The model under review builds one solid part; all positions refer to its coordinate system, in mm. A direction names the side the tool comes from. Give positions to 0.01 mm unless a question says otherwise; leave off trailing zeros. Order: outer loops, then holes, each group sorted by start corner. A loop starts at its lowest first (then second) coordinate and runs counter-clockwise, first axis right, second up. Notation, with made-up numbers: (40, -34) - (53, -34) arc R36 cw to (53, 3) - close; hole circle Ø1 at (-17.5, -38.75). An arc over 180 degrees is marked (long way). Use CSV: the item, a comma, the result in double quotes. Start each with the question number.
1. Take a section at A-A, the plane z = 31.5. State the section outline as (x, y) points, then the cut area to 3 significant figures.
2. Take a section at C-C, the plane x = -126.5. State the section outline as (y, z) points.
3. Machinability: for faces 5 (the flat face through (-102, 0, 10)), 6 (the flat face through (-152.89, 4, 31)), which of the approach directions +Z, -Z, +X, -X, +Y, -Y give a long, thin tool a straight path to every point of the face, cutting with its end or side? Answer none if there is none.
4. Draft analysis for pull direction X (two halves, no side actions). For faces 1 (the flat face through (-118, 10, 52)), 2 (the flat face through (-103, 4, 10.186)), 3 (the flat face through (-49.89, 5, 31)), 4 (the flat face through (-102, 9, 52)), state which applies: released by +X, released by -X, zero draft, split by the parting line, or undercut.
5. Take a section at B-B, the plane y = 6. State the section outline as (x, z) points, then the cut area to 3 significant figures.
6. To check wall thickness, follow line 1 (Z direction, x = -131, y = 3.75); line 2 (X direction, y = 0.5, z = 34). State the ranges of each line that lie inside material, in increasing order. Write a range as [from, to].
```python
from build123d import *

# Parameters (mm, degrees)
F0_W     = 104
F0_H     = 44
F0_W_2   = 100
F0_H_2   = 40
F1_DEPTH = 10
F2_T     = -1
F3_DEPTH = 25


with BuildPart() as f1:
    # F0 (on Front) → F1 (new body)
    with BuildSketch(Plane.XZ):
        with Locations((-101.889864, 31.185937)):
            Rectangle(F0_W, F0_H)
        with Locations((-101.889864, 31.185937)):
            Rectangle(F0_W_2, F0_H_2, mode=Mode.SUBTRACT)
        with Locations((-101.889864, 31.185937)):
            Rectangle(F0_W_2, F0_H_2)
    extrude(amount=-F1_DEPTH)

    # F2
    f2_openings = [f1.faces().sort_by_distance(p)[0] for p in [
        (-101.889864, 0, 31.185937),
    ]]
    offset(amount=F2_T, openings=f2_openings)

    # F0 (on Front) → F3 (cut)
    with BuildSketch(Plane.XZ):
        with Locations((-101.889864, 31.185937)):
            Rectangle(F0_W_2, F0_H_2)
    extrude(amount=-F3_DEPTH, mode=Mode.SUBTRACT)


solid = f1.part
```
Determined:
1,outline,"(-153.89, 0) - (-152.89, 0) - (-152.89, 9) - (-151.89, 9) - (-151.89, 10) - (-153.89, 10) - close; (-51.89, 9) - (-50.89, 9) - (-50.89, 0) - (-49.89, 0) - (-49.89, 10) - (-51.89, 10) - close"
1,area,"22.0 mm²"
2,outline,"(0, 9.19) - (10, 9.19) - (10, 11.19) - (9, 11.19) - (9, 10.19) - (0, 10.19) - close; (0, 52.19) - (9, 52.19) - (9, 51.19) - (10, 51.19) - (10, 53.19) - (0, 53.19) - close"
3,face 5,"+Z, -Z, +X, -X, -Y"
3,face 6,"-Y"
4,face 1,"zero draft"
4,face 2,"undercut"
4,face 3,"released by +X"
4,face 4,"undercut"
5,outline,"(-153.89, 9.19) - (-49.89, 9.19) - (-49.89, 53.19) - (-153.89, 53.19) - close; hole (-152.89, 10.19) - (-50.89, 10.19) - (-50.89, 52.19) - (-152.89, 52.19) - close"
5,area,"292 mm²"
6,line 1,"z = [9.19, 10.19], [52.19, 53.19]"
6,line 2,"x = [-153.89, -152.89], [-50.89, -49.89]"
